Job drawing, mm, ordinate dimensions from the low corner. One solid piece. A direction names the side the tool comes from. Give positions to 0.01 mm unless a question says otherwise; leave off trailing zeros. Write each loop counter-clockwise with the first axis right and the second up, starting at its lowest first coordinate (ties: lowest second). Pieces come first, ordered by that corner, then holes. Notation, with made-up numbers: M 43,4.5 L 64,4.5 A14 ccw 64,19.5 Z; hole C 85.25,25 d5. An arc over 180 degrees is marked long. Use CSV: the item, a comma, the result in double quotes. Start each with the question number.
Item 1: Cut at B-B (x = 13.5). List the corners of the cut face in (y, z), then the cut area to 3 significant figures.
Item 2: Cut at A-A (z = 41). List the corners of the cut face in (x, y), then the cut area to 3 significant figures.
Item 3: Drill centre lines: line 1 (Y direction, x = 3.5, z = 74.5); line 2 (X direction, y = 33, z = 18). Where is each one in solid material? Low to high. Write a range as [from, to].
Item 4: Which spindle directions (+Z, -Z, +X, -X, +Y, -Y) get a long thin tool onto all of the face, cutting with end or side? Do the marked faces 1, 2 and 3. Say none if no direction does.
Item 5: Pin check, flat tips, straight feed: pin 1 (7.5 mm diameter, centred on x = 10, z = 50.5, fed in from +Y); pin 2 (4.5 mm diameter, centred on x = 5.5, z = 44.5, fed in from -Y); pin 3 (2 mm diameter, centred on y = 1.5, z = 33.5, fed in from -X). Stop position of each tip, or through.
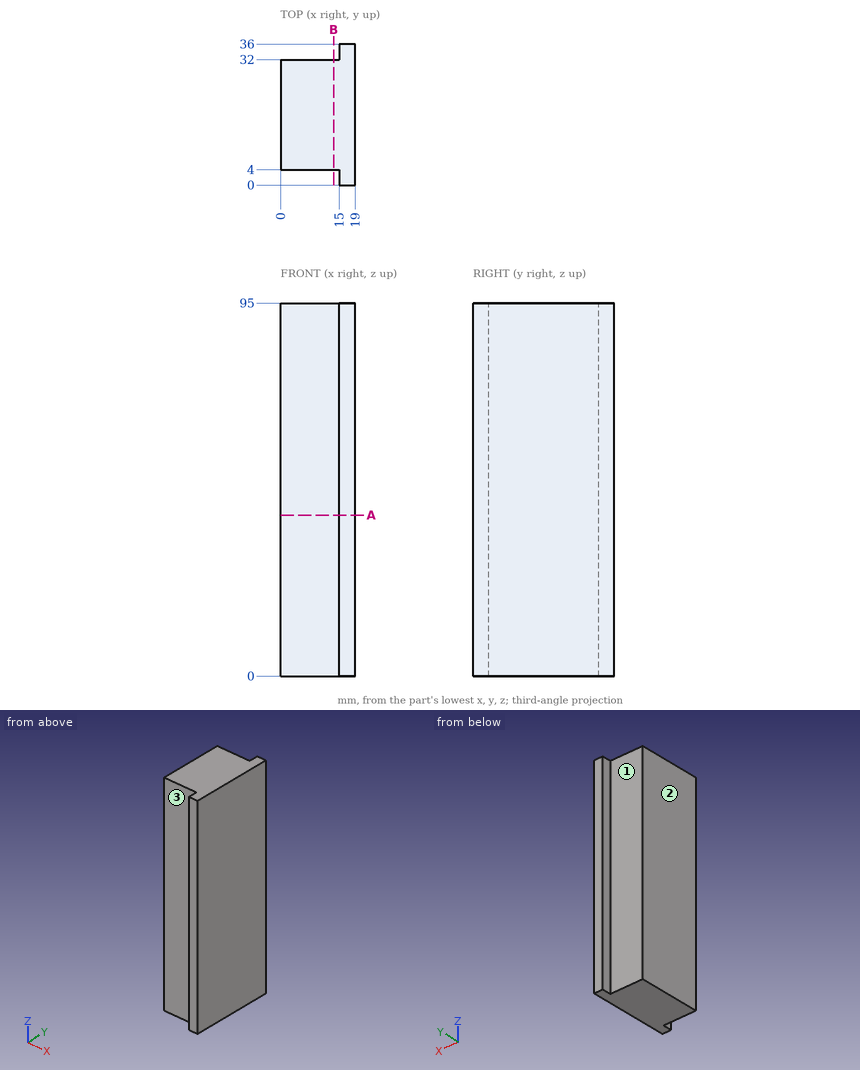
Worked answers:
1,outline,"M 4,0 L 32,0 L 32,95 L 4,95 Z"
1,area,"2,660 mm^2"
2,outline,"M 0,4 L 15,4 L 15,0 L 19,0 L 19,36 L 15,36 L 15,32 L 0,32 Z"
2,area,"564 mm^2"
3,line 1,"y = [4, 32]"
3,line 2,"x = [15, 19]"
4,face 1,"+Z, -Z, -X, +Y"
4,face 2,"+Z, -Z, -X, +Y, -Y"
4,face 3,"+Z, -Z, -X, -Y"
5,pin 1,"stops at y = 32"
5,pin 2,"stops at y = 4"
5,pin 3,"stops at x = 15"
